Check sheet for the modelled part. Datum: model origin and axes. Units: mm. Face numbers are marked on the shaded views. Round coordinates to 2 decimals unless told otherwise and drop trailing zeros. Write each loop counter-clockwise with the first axis right and the second up, starting at its lowest first coordinate (ties: lowest second). Pieces come first, ordered by that corner, then holes. Notation, with made-up numbers: (78, 9) -> (118, 9) arc R18 ccw to (118, 22) -> close; hole circle Ø6 at (-19.75, 71). An arc over 180 degrees is marked (long way). Answer as a JSON object with one key per item and string values. Group by question number.
Autodesk Inventor part; units mm, degrees
ref_plane "YZ Plane" through (0, 0, 0) normal (1, 0, 0) x (0, 1, 0)
ref_plane "XZ Plane" through (0, 0, 0) normal (0, 1, 0) x (-1, 0, 0)
ref_plane "XY Plane" through (0, 0, 0) normal (0, 0, 1) x (1, 0, 0)
sketch "Sketch1" plane through (0, 0, 0) normal (0, 0, 1) x (1, 0, 0)
  line L0 (-8, 32) -> (8, 32)
  line L1 (8, 32) -> (8, -32)
  line L2 (8, -32) -> (-8, -32)
  line L3 (-8, -32) -> (-8, 32)
  point P0 (0, 0)
  dimension "d0" = 16
  dimension "d1" = 64
  dimension "d2" = 8
  dimension "d3" = 32
extrude "Extrusion1" add sketch "Sketch1" along normal blind 9.6
shell "Shell1" thickness 1.5 removed faces 1 at (-2.6667, 10.6667, 0)
sketch "Sketch2" plane through (0, 0, 9.6) normal (0, 0, 1) x (1, 0, 0)
  circle A0 centre (4, -28) radius 2.5
  line L0 (8, 32) -> (8, -32)
  line L1 (8, -32) -> (-8, -32)
  dimension "d7" = 5
  dimension "d10" = 4
  dimension "d11" = 4
extrude "Extrusion2" add sketch "Sketch2" along normal blind 1.6
sketch "Sketch3" plane through (6.5, -30.5, 8.1) normal (0, 0, -1) x (-1, 0, 0)
  circle A0 centre (2.5, 2.5) radius 2.5
  circle A1 centre (2.5, 2.5) radius 1.2
  point P0 (6.5, 30.5)
  dimension "d18" = 2.4
extrude "Extrusion3" cut sketch "Sketch3" against normal blind 1.6 contours A1
pattern_linear "Rectangular Pattern1" count 8 spacing 8 along (0, 1, 0) count 2 spacing 8 along (-1, 0, 0) of "Extrusion2", "Extrusion3"
sketch "Sketch4" plane through (6.5, -30.5, 8.1) normal (0, 0, -1) x (-1, 0, 0)
  circle A0 centre (2.5, 10.5) radius 1.2
  circle A1 centre (2.5, 2.5) radius 1.2
  line L0 (0, 61) -> (0, 0)
  line L1 (0, 0) -> (13, 0)
  circle A2 centre (6.5, 6.5) radius 3.15
  circle A3 centre (6.5, 6.5) radius 2.5
  point P0 (6.5, 30.5)
  dimension "d21" = 6.5
  dimension "d22" = 6.5
  dimension "d23" = 10.5
  dimension "d24" = 2.5
  dimension "d25" = 5
  dimension "d26" = 6.3
extrude "Extrusion4" add sketch "Sketch4" along normal up to surface (8.1 mm away) contours A2
pattern_linear "Rectangular Pattern2" count 7 spacing 8 along (0, 1, 0) of "Extrusion4"
equation "\"d0\" = 0.8 * WIDTH"
equation "\"d1\" = 0.8 * LENGTH"
equation "\"d21\" = 0.5 * d23 + 0.5 * d24"
equation "\"d22\" = d21"
equation "\"WIDTH\" = 2"
properties part number "3007" material "Steel"
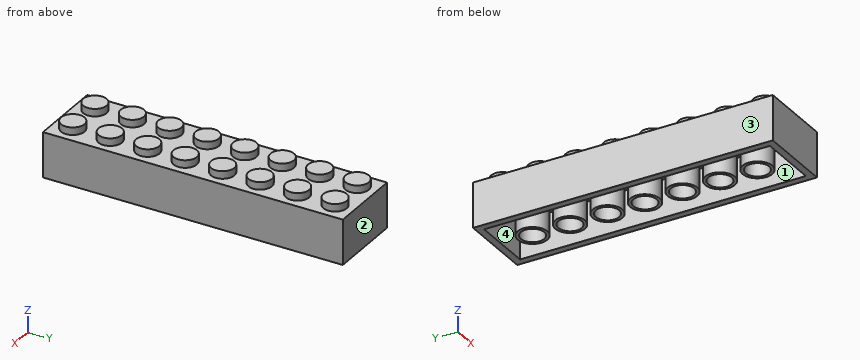
(1) Section check A-A on z = 7.25. State how many separate pieces and enclosed holes the cut face has, then the cut area to 3 significant figures.
(2) Go/stop test with flat-tipped pins: pin 1 Ø1.4 at (x, y) = (-4, 12) entering from -Z; pin 2 Ø1.5 at (x, y) = (-0.5, -25) entering from -Z; pin 3 Ø5.5 at (x, y) = (0.5, 7) entering from -Z; pin 4 Ø1.5 at (x, y) = (2, 23.5) entering from +Z. Record where each tip stops, or that it passes through.
(3) Scan lines: line 1 along Y through (x, z) = (-5.5, 1.5); line 2 along Z through (x, y) = (0.5, -27.5); line 3 along X through (y, z) = (-5, 10.25). Record each from-to range of solid material in increasing order.
(4) Release check for a two-part mould opening along X. For the marked faces 1, 2, 3 and 4 record: pulls with the +X half, pulls with the -X half, needs draft (parallel to the pull), parting line crosses it, or undercut.
(5) Section check B-B on y = -24. Record the cut outline in (x, z), then the cut area to 3 significant figures.
Data:
{
 "1": {"separate pieces": "8", "enclosed holes": "8", "area": "312 mm²"},
 "2": {"pin 1": "stops at z = 9.7", "pin 2": "stops at z = 8.1", "pin 3": "stops at z = 0", "pin 4": "stops at z = 9.6"},
 "3": {"line 1": "y = -32 to -30.5, 30.5 to 32", "line 2": "z = 8.1 to 9.6", "line 3": "x = -6.29 to -1.71, 1.71 to 6.29"},
 "4": {"face 1": "undercut", "face 2": "needs draft", "face 3": "pulls with the -X half", "face 4": "undercut"},
 "5": {"outline": "(-8, 0) -> (-6.5, 0) -> (-6.5, 8.1) -> (-3.15, 8.1) -> (-3.15, 0) -> (-2.5, 0) -> (-2.5, 8.1) -> (2.5, 8.1) -> (2.5, 0) -> (3.15, 0) -> (3.15, 8.1) -> (6.5, 8.1) -> (6.5, 0) -> (8, 0) -> (8, 9.6) -> (-8, 9.6) -> close", "area": "58.8 mm²"}
}
